```python
from build123d import *

# Parameters (mm, degrees)
F0_R     = 13.1240937351
F1_DEPTH = 25.4
F2_SIZE  = 5.08
F3_R     = 12.3312643235
F4_DEPTH = 25.4
F5_DEPTH = 52.578
F6_R     = 12.3312643235


with BuildPart() as f1:
    # F0 (on Top) → F1 (new body)
    with BuildSketch(Plane.XY):
        with Locations((6.1321523972, 1.8493796233)):
            Circle(F0_R)
    extrude(amount=F1_DEPTH)

    # F2
    f2_edges = [f1.edges().sort_by_distance(p)[0] for p in [
        (-6.991941, 1.84938, 25.4),
        (-6.991941, 1.84938, 0),
    ]]
    chamfer(f2_edges, length=F2_SIZE)

    # F3
    f3_edges = [f1.edges().sort_by_distance(p)[0] for p in [
        (-1.911941, 1.84938, 25.4),
    ]]
    fillet(f3_edges, radius=F3_R)

    # F4 (add): a face of the model
    f4_faces = [f1.faces().sort_by_distance(p)[0] for p in [
        (6.1321523972, 1.8493796233, 25.4),
    ]]
    extrude(f4_faces, amount=F4_DEPTH)

    # F5 (add): a face of the model
    f5_faces = [f1.faces().sort_by_distance(p)[0] for p in [
        (6.1321523972, 1.8493796233, 50.8),
    ]]
    extrude(f5_faces, amount=F5_DEPTH)

    # F6
    f6_edges = [f1.edges().sort_by_distance(p)[0] for p in [
        (-1.911941, 1.84938, 0),
    ]]
    fillet(f6_edges, radius=F6_R)


solid = f1.part
```
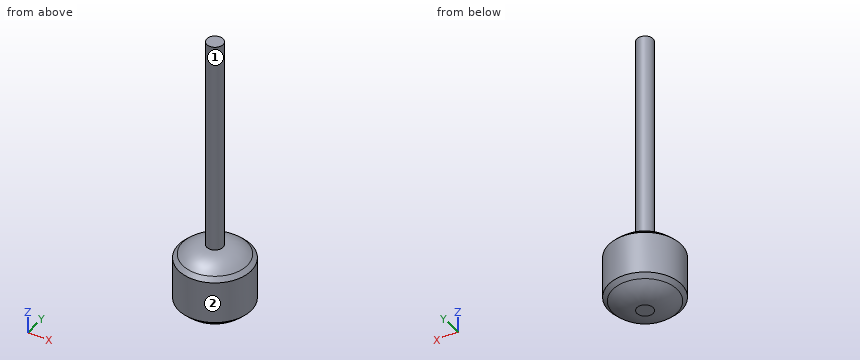
CAD build for the part. Positions are in the model's coordinates, mm. Face numbers are marked on the shaded views. A direction names the side the tool comes from. Coordinates: 2 decimals unless noted, no trailing zeros. Order: outer loops, then holes, each group sorted by start corner. A loop starts at its lowest first (then second) coordinate and runs counter-clockwise, first axis right, second up. Notation, with made-up numbers: (17, -25) - (64, -25) arc R25 cw to (64, -6) - close; hole circle Ø5 at (25, 7.5). An arc over 180 degrees is marked (long way). Use a Markdown table: item, result. Add a question column.
(1) Which spindle directions (+Z, -Z, +X, -X, +Y, -Y) get a long thin tool onto all of the face, cutting with end or side? Do the marked faces 1 and 2. Say none if no direction does.
(2) Saw through at B-B (z = 11). Give the cut face in (x, y), then the cut area to 3 significant figures.
(3) Saw through at A-A (z = 57). Give the cut face in (x, y), then the cut area to 3 significant figures.
(4) Flat gauge pins, fed straight in: pin 1 (2 mm diameter, centred on y = 8, z = 21.5, fed in from -X); pin 2 (10 mm diameter, centred on y = -1, z = 78.5, fed in from -X); pin 3 (10 mm diameter, centred on x = 1, y = -4.5, fed in from -Z). Where does each tip first touch, or does it go through?
(5) Drill centre lines: line 1 along Y through (x, z) = (1.5, 12); line 2 along Y through (x, z) = (11.5, 21); line 3 along X through (y, z) = (11, 6). Where is each one in solid material? Low to high. Write a range as [from, to].
Solved:
| question | item | result |
|---|---|---|
| 1 | face 1 | +Z |
| 1 | face 2 | +Z, -Z |
| 2 | outline | circle Ø26.25 at (6.13, 1.85) |
| 2 | area | 541 mm² |
| 3 | outline | circle Ø5.87 at (6.13, 1.85) |
| 3 | area | 27.1 mm² |
| 4 | pin 1 | stops at x = -5.37 |
| 4 | pin 2 | stops at x = 3.2 |
| 4 | pin 3 | stops at z = 0 |
| 5 | line 1 | y = [-10.43, 14.13] |
| 5 | line 2 | y = [-9.38, 13.08] |
| 5 | line 3 | x = [-3.28, 15.54] |
